```python
from build123d import *

# Parameters (mm, degrees)
BOSS_EXTRUDE1_DEPTH = 9
CHAMFER1_SIZE       = 5
SKETCH2_R           = 15
CUT_EXTRUDE1_DEPTH  = 606.180442557


with BuildPart() as part:
    # Sketch1 → Boss-Extrude1 (new body)
    with BuildSketch(Plane(origin=(0, 0, 0), x_dir=(1, 0, 0), z_dir=(0, 1, 0))):
        with BuildLine():
            ThreePointArc((-54.052143505, 516.045456082), (0, 550), (54.052143505, 516.045456082))
            ThreePointArc((54.052143505, 516.045456082), (212.411110101, 45.380156813), (249.928432165, -449.792375526))
            ThreePointArc((249.928432165, -449.792375526), (239.970710869, -480.073057321), (215.909090909, -500.980337113))
            ThreePointArc((215.909090909, -500.980337113), (0, -550), (-215.909090909, -500.980337113))
            ThreePointArc((-215.909090909, -500.980337113), (-239.970710869, -480.073057321), (-249.928432165, -449.792375526))
            ThreePointArc((-249.928432165, -449.792375526), (-212.411110101, 45.380156813), (-54.052143505, 516.045456082))
        make_face()
    extrude(amount=-BOSS_EXTRUDE1_DEPTH)

    # Chamfer1
    chamfer1_edges = [part.edges().sort_by_distance(p)[0] for p in [
        (0, 0, -550),
        (212.411110101, 0, -45.380156813),
        (239.970710869, 0, 480.073057321),
        (0, 0, 550),
        (-239.970710869, 0, 480.073057321),
        (-212.411110101, 0, -45.380156813),
    ]]
    chamfer(chamfer1_edges, length=CHAMFER1_SIZE)

    # Sketch2 → Cut-Extrude1 (cut, through all)
    with BuildSketch(Plane(origin=(0, 0, 0), x_dir=(1, 0, 0), z_dir=(0, 1, 0))):
        with Locations(Location((0, 105, 0), (0, 0, 270))):
            Circle(SKETCH2_R)
        with Locations(Location((0, -120, 0), (0, 0, 270))):
            Circle(SKETCH2_R)
    extrude(amount=-CUT_EXTRUDE1_DEPTH, mode=Mode.SUBTRACT)


solid = part.part
```
Source: CAD feature listing. Evaluate the final solid. Frame: model axes, mm. Coordinates: 2 decimals unless noted, no trailing zeros. Loops run counter-clockwise (first coordinate to the right, second up) from the corner with the lowest first, then second, coordinate; pieces in that order, holes last. Notation, with made-up numbers: (-37.75, 1.5) -> (-6.75, 1.5) arc R10 ccw to (-6.75, 9.5) -> close; hole circle Ø6 at (-17, 36.25). An arc over 180 degrees is marked (long way). One line per item, written item: value. Start each with the question number.
Q1. Line query: line 1 along X through (y, z) = (-6.5, -105); line 2 along X through (y, z) = (-5, 120); line 3 along X through (y, z) = (-6.5, 365.5). Output: solid intervals per line, ascending.
Q2. Section query B-B, the plane y = -6.75. Return the cut outline in (x, z).
Q3. Mould query, pull axis X, two halves, no side actions, for faces 1 (the face through (240.219, -6.972, 479.696)), 2 (the face through (-239.72, -6.97, 480.45)), 3 (the face through (12.65, -4.44, -96.94)). Classes: pulls with the +X half, pulls with the -X half, needs draft (parallel to the pull), parting line crosses it, or undercut.
Q4. Contact query for flat-ended pins moving along their axis: P1, Ø5, axis at y = -2.5, z = -158, coming from the -X side; P2, Ø2, axis at x = -155, y = -6, coming from the +Z side; P3, Ø1.5, axis at y = -2, z = 268.5, coming from the +X side. Output: stop coordinate, or through.
Q5. Section query A-A, the plane x = 0. Return the cut outline in (y, z).
Results:
1. line 1: -199.37 to -15, 15 to 199.37
1. line 2: -238.8 to -15, 15 to 238.8
1. line 3: -252.27 to 252.27
2. outline: (-249.93, 449.79) arc R2000 ccw to (-54.05, -516.05) arc R60 ccw to (54.05, -516.05) arc R2000 ccw to (249.93, 449.79) arc R60 ccw to (215.91, 500.98) arc R500 ccw to (-215.91, 500.98) arc R60 ccw to start; hole circle Ø30 at (0, -105); hole circle Ø30 at (0, 120)
3. face 1: pulls with the +X half
3. face 2: pulls with the -X half
3. face 3: undercut
4. P1: x = -186.24
4. P2: z = 525.69
4. P3: x = 248.31
5. outline: (-9, -550) -> (-5, -550) -> (0, -545) -> (0, -120) -> (-9, -120) -> close; (-9, -90) -> (0, -90) -> (0, 105) -> (-9, 105) -> close; (-9, 135) -> (0, 135) -> (0, 545) -> (-5, 550) -> (-9, 550) -> close
